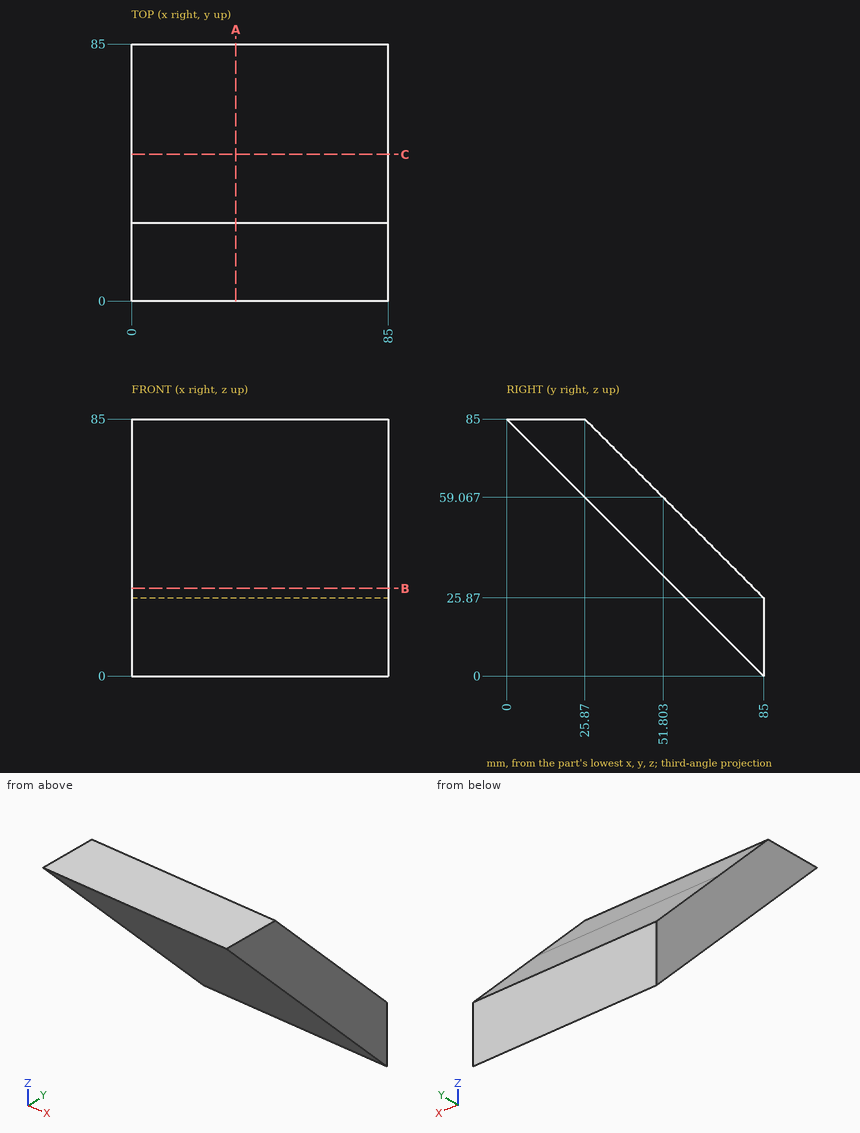
Part print with two shaded views. Sizes in mm from the minimum x, y, z corner. Coordinates: 2 decimals unless noted, no trailing zeros. Loops run counter-clockwise (first coordinate to the right, second up) from the corner with the lowest first, then second, coordinate; pieces in that order, holes last. Notation, with made-up numbers: M 3.25,78.5 L 43.25,78.5 A28 cw 43.25,102.5 Z; hole C 81,-13 d5. An arc over 180 degrees is marked long. Use CSV: the item, a comma, the result in double quotes. Start each with the question number.
1. Flat gauge pins, fed straight in: pin 1 (3 mm diameter, centred on x = 11, z = 42.5, fed in from -Y); pin 2 (3 mm diameter, centred on x = 56.5, z = 26.5, fed in from +Y); pin 3 (1 mm diameter, centred on x = 14.5, y = 73.5, fed in from -Z); pin 4 (12 mm diameter, centred on x = 14.5, y = 71.5, fed in from -Z). Where does each tip first touch, or does it go through?
2. Band-saw the part on C-C, the plane y = 48.5. List the corners of the cut face in (x, z), then the cut area to 3 significant figures.
3. Band-saw the part on B-B, the plane z = 29. List the corners of the cut face in (x, y), then the cut area to 3 significant figures.
4. Band-saw the part on A-A, the plane x = 34.5. List the corners of the cut face in (y, z).
5. Probe probe 1 along Z at (x, y) = (60.5, 42.5); probe 2 along Z at (x, y) = (28, 81.5); probe 3 along Y at (x, z) = (35.5, 9). List the from-to ranges inside material, lowest first. Write a range as [from, to].
Entries:
1,pin 1,"stops at y = 41"
1,pin 2,"stops at y = 85"
1,pin 3,"stops at z = 11"
1,pin 4,"stops at z = 7.5"
2,outline,"M 0,36.5 L 85,36.5 L 85,62.37 L 0,62.37 Z"
2,area,"2,200 mm2"
3,outline,"M 0,56 L 85,56 L 85,81.87 L 0,81.87 Z"
3,area,"2,200 mm2"
4,outline,"M 0,85 L 85,0 L 85,25.87 L 25.87,85 Z"
5,probe 1,"z = [42.5, 68.37]"
5,probe 2,"z = [3.5, 29.37]"
5,probe 3,"y = [76, 85]"
